Can you work these out from the model? Positions are in its coordinate system, mm. A direction names the side the tool comes from. Give positions to 0.01 mm unless a question says otherwise; leave off trailing zeros. Order: outer loops, then holes, each group sorted by start corner. A loop starts at its lowest first (then second) coordinate and runs counter-clockwise, first axis right, second up. Notation, with made-up numbers: M 12.5,-17.75 L 21.5,-17.75 A11 cw 21.5,-0.75 Z; hole C -30.5,42 d5. An arc over 180 degrees is marked long. Write each question's results on one line, items separated by ' | '.
from build123d import *

# Parameters (mm, degrees)
F0_R     = 4.142858
F1_DEPTH = 12.7
F3_DEPTH = 36.068
F4_DEPTH = 7.874
F5_DEPTH = 7.874
F6_DEPTH = 12.7
F8_DEPTH = 38.354


with BuildPart() as f1:
    # F0 (on Front) → F1 (new body, symmetric)
    with BuildSketch(Plane.XZ):
        Polygon((23.873951, 16.499758), (-42.309441, 16.499758), (-64.985082, -8.388145), (23.873951, -8.388145), align=None)
        with Locations((-27.192343, 4.516693)):
            Circle(F0_R, mode=Mode.SUBTRACT)
        with BuildLine():
            ThreePointArc((1.935726, 8.94121), (3.594917, 9.242078), (5.254109, 8.94121))
            ThreePointArc((5.254109, 8.94121), (7.478832, 7.208249), (8.320303, 4.516693))
            ThreePointArc((8.320303, 4.516693), (7.395697, 1.708964), (4.983711, 0))
            ThreePointArc((4.983711, 0), (3.594917, -0.208692), (2.206124, 0))
            ThreePointArc((2.206124, 0), (-1.128308, 4.373854), (1.935726, 8.94121))
        make_face(mode=Mode.SUBTRACT)
        with BuildLine():
            ThreePointArc((8.320303, 4.516693), (7.478832, 7.208249), (5.254109, 8.94121))
            Line((5.254109, 8.94121), (1.935726, 8.94121))
            ThreePointArc((1.935726, 8.94121), (-1.128308, 4.373854), (2.206124, 0))
            Line((2.206124, 0), (4.983711, 0))
            ThreePointArc((4.983711, 0), (7.395697, 1.708964), (8.320303, 4.516693))
        make_face()
        with Locations((-27.192343, 4.516693)):
            Circle(F0_R)
        with BuildLine():
            Line((4.983711, 0), (2.206124, 0))
            ThreePointArc((2.206124, 0), (3.594917, -0.208692), (4.983711, 0))
        make_face()
        with BuildLine():
            Line((1.935726, 8.94121), (5.254109, 8.94121))
            ThreePointArc((5.254109, 8.94121), (3.594917, 9.242078), (1.935726, 8.94121))
        make_face()
    extrude(amount=F1_DEPTH, both=True)

    # F2 (on Front) → F3 (cut)
    with BuildSketch(Plane.XZ):
        with BuildLine():
            Line((1.877148, 7.4168), (-27.933743, 7.4168))
            ThreePointArc((-27.933743, 7.4168), (-31.642143, 3.7084), (-27.933743, 0))
            Line((-27.933743, 0), (0, 0))
            ThreePointArc((0, 0), (5.702478, 2.502684), (1.877148, 7.4168))
        make_face()
    extrude(amount=F3_DEPTH, mode=Mode.SUBTRACT)

    # F0 (on Front) → F4 (join, symmetric)
    with BuildSketch(Plane.XZ):
        Polygon((-42.309441, 35.119597), (-42.309441, 16.499758), (23.873951, 16.499758), (23.873951, 34.566533), align=None)
    extrude(amount=F4_DEPTH, both=True)

    # F0 (on Front) → F5 (join, symmetric)
    with BuildSketch(Plane.XZ):
        Polygon((-41.998268, 53.736836), (-42.309441, 35.119597), (23.873951, 34.566533), (24.175882, 52.630785), align=None)
    extrude(amount=F5_DEPTH, both=True)

    # F0 (on Front) → F6 (join, symmetric)
    with BuildSketch(Plane.XZ):
        Polygon((-64.254817, 79.000216), (-41.998268, 53.736836), (24.175882, 52.630785), (24.591806, 77.515212), align=None)
        with Locations((-26.683021, 65.465591)):
            Circle(F0_R, mode=Mode.SUBTRACT)
        with BuildLine():
            ThreePointArc((8.825325, 64.951077), (7.961227, 62.22716), (5.684958, 60.49945))
            ThreePointArc((5.684958, 60.49945), (4.02097, 60.226352), (2.367037, 60.554907))
            ThreePointArc((2.367037, 60.554907), (-0.620239, 65.17283), (2.786823, 69.490349))
            ThreePointArc((2.786823, 69.490349), (4.17891, 69.675802), (5.564021, 69.44393))
            ThreePointArc((5.564021, 69.44393), (7.924048, 67.726948), (8.825325, 64.951077))
        make_face(mode=Mode.SUBTRACT)
    extrude(amount=F6_DEPTH, both=True)

    # F7 (on Front) → F8 (cut)
    with BuildSketch(Plane.XZ):
        Polygon((-27.697399, 60.589042), (1.984779, 60.589042), (3.067527, 69.898891), (-27.697399, 69.898891), align=None)
    extrude(amount=F8_DEPTH, mode=Mode.SUBTRACT)


solid = f1.part
(1) Imagine slicing it at C-C, the plane x = -48.5. Write out the boundary of the cut face in (y, z), plus the area to 3 significant figures.
Data:
outline: M -12.7,-8.39 L 12.7,-8.39 L 12.7,9.71 L -12.7,9.71 Z; M -12.7,61.12 L 12.7,61.12 L 12.7,78.74 L -12.7,78.74 Z | area: 907 mm2
(2) I need wall thicknesses on L1, parallel to Z at x = -9.5, y = -3.5; L2, parallel to X at y = 1.75, z = 64; L3, parallel to Z at x = -24.5, y = -5. Which ranges of each line are inside material? Lowest first, please. Write a range as from..to.
Data:
L1: z = -8.39..0, 7.42..60.59, 69.9..78.09 | L2: x = -51.04..-30.56, -22.81..-0.53, 8.73..24.37 | L3: z = -8.39..0, 7.42..60.59, 69.9..78.34
(3) Will these pins go through, and if not, where does the flat tip stop? P1, Ø4, axis at x = -16, y = -3.5, coming from the +Z side; P2, Ø0.5, axis at y = -5.5, z = 69.5, coming from the +X side; P3, Ø3, axis at x = -41, z = 46.5, coming from the +Y side.
Data:
P1: stops at z = 78.23 | P2: stops at x = 24.46 | P3: stops at y = 7.87
(4) Imagine slicing it at B-B, the plane z = 68. Write out the boundary of the cut face in (x, y).
Data:
outline: M -54.56,-12.7 L -29.96,-12.7 L -29.96,12.7 L -54.56,12.7 Z; M -23.41,0 L 0.49,0 L 0.49,12.7 L -23.41,12.7 Z; M 7.71,-12.7 L 24.43,-12.7 L 24.43,12.7 L 7.71,12.7 Z
(5) Imagine slicing it at D-D, the plane x = -33. Write out the boundary of the cut face in (y, z).
Data:
outline: M -12.7,-8.39 L 12.7,-8.39 L 12.7,16.5 L 7.87,16.5 L 7.87,53.59 L 12.7,53.59 L 12.7,78.48 L -12.7,78.48 L -12.7,53.59 L -7.87,53.59 L -7.87,16.5 L -12.7,16.5 Z
(6) For faces 4 (the face through (-53.49, -0.18, 4.23)), 5 (the face through (-9, 10, 16.5)), 6 (the face through (-31.64, -6.26, 3.79)), which set-ups out of +Z, -Z, +X, -X, +Y, -Y let a thin tool reach every point of the face, with its end or its side?
Data:
face 4: -X, +Y, -Y | face 5: +X, -X, +Y | face 6: -Y
(7) We'd pull the mould along Z, two halves only. Please class faces 1 (the face through (23.874, 0, 8)), 2 (the face through (-21, 0, -8.388)), 3 (the face through (-13, 0, 65)): +Z half, -Z half, draft (parallel to the pull), parting line (faces both ways), or undercut.
Data:
face 1: draft | face 2: -Z half | face 3: undercut
(8) Imagine slicing it at A-A, the plane y = -9.75. Write out the boundary of the cut face in (x, z), plus the area to 3 significant figures.
Data:
outline: M -64.99,-8.39 L 23.87,-8.39 L 23.87,16.5 L -42.31,16.5 Z; M -64.25,79 L -42,53.74 L 24.18,52.63 L 24.59,77.52 Z; hole M -27.93,0 L 0,0 A3.95 ccw long 1.88,7.42 L -27.93,7.42 A3.71 ccw Z; hole M -27.7,60.59 L 1.98,60.59 L 2,60.72 A4.73 ccw 2.37,60.55 A4.73 ccw 5.68,60.5 A4.73 ccw 8.83,64.95 A4.73 ccw 5.56,69.44 A4.73 ccw 3.03,69.55 L 3.07,69.9 L -27.7,69.9 L -27.7,69.48 A4.14 ccw -27.7,61.45 Z | area: 3,240 mm2
